from build123d import *

# Parameters (mm, degrees)
SKETCH014_R          = 2.2
PAD013_DEPTH         = 1.8
SKETCH015_W          = 30
SKETCH015_H          = 6
PAD014_DEPTH         = 0.75
FILLET004_R          = 0.7499
SKETCH016_W          = 25
SKETCH016_H          = 15
SKETCH017_W          = 6.5
SKETCH017_H          = 15
LOFT_PLACEMENT_ANGLE = 180
PAD015_DEPTH         = 3.25
SKETCH019_R          = 1.75
POCKET003_DEPTH      = 6.5


with BuildPart() as fillet004:
    # Sketch014 → Pad013 (new body)
    with BuildSketch(Plane.XZ):
        with BuildLine():
            Line((-25.5, 7.5), (25.5, 7.5))
            ThreePointArc((27.5, 5.5), (26.914214, 6.914214), (25.5, 7.5))
            Line((27.5, 5.5), (27.5, -5.5))
            ThreePointArc((25.5, -7.5), (26.914214, -6.914214), (27.5, -5.5))
            Line((25.5, -7.5), (-25.5, -7.5))
            ThreePointArc((-27.5, -5.5), (-26.914214, -6.914214), (-25.5, -7.5))
            Line((-27.5, -5.5), (-27.5, 5.5))
            ThreePointArc((-25.5, 7.5), (-26.914214, 6.914214), (-27.5, 5.5))
        make_face()
        with Locations((-20, 0)):
            Circle(SKETCH014_R, mode=Mode.SUBTRACT)
        with Locations((20, 0)):
            Circle(SKETCH014_R, mode=Mode.SUBTRACT)
    extrude(amount=PAD013_DEPTH)

    # Sketch015 → Pad014 (new body)
    with BuildSketch(Plane.XZ.offset(1.8)):
        Rectangle(SKETCH015_W, SKETCH015_H)
    extrude(amount=PAD014_DEPTH)

    # Fillet004
    fillet004_edges = [fillet004.edges().sort_by_distance(p)[0] for p in [
        (-15, -2.55, 0),
        (0, -2.55, 3),
        (15, -2.55, 0),
        (0, -2.55, -3),
    ]]
    fillet(fillet004_edges, radius=FILLET004_R)


with BuildPart() as fusion001:
    # Sketch016 → Loft section 0
    with BuildSketch(Plane.XZ):
        Rectangle(SKETCH016_W, SKETCH016_H)
    # Sketch017 → Loft section 1
    with BuildSketch(Plane.XZ.offset(15)):
        Rectangle(SKETCH017_W, SKETCH017_H)
    loft(ruled=True)


with BuildPart() as fusion001_1:
    # Loft placement: moved
    add(fusion001.part.rotate(Axis((0, 0, 0), (0, 0, 1)), LOFT_PLACEMENT_ANGLE))

    # Fusion001: union Fillet004
    add(fillet004.part)


with BuildPart() as fusion002:
    # Sketch018 → Pad015 (new body, symmetric)
    with BuildSketch(Plane(origin=(0, 15, 0), x_dir=(0, 1, 0), z_dir=(1, 0, 0))):
        with BuildLine():
            Line((0, 7.5), (9, 7.5))
            ThreePointArc((9, -7.5), (16.5, 0), (9, 7.5))
            Line((9, -7.5), (0, -7.5))
            Line((0, -7.5), (0, 7.5))
        make_face()
    extrude(amount=PAD015_DEPTH, both=True)

    # Sketch019 → Pocket003 (cut)
    with BuildSketch(Plane(origin=(3.25, 15, 0), x_dir=(0, 1, 0), z_dir=(1, 0, 0))):
        with Locations((9, 0)):
            Circle(SKETCH019_R)
    extrude(amount=-POCKET003_DEPTH, mode=Mode.SUBTRACT)

    # Fusion002: union Fusion001
    add(fusion001_1.part)


solid = fusion002.part
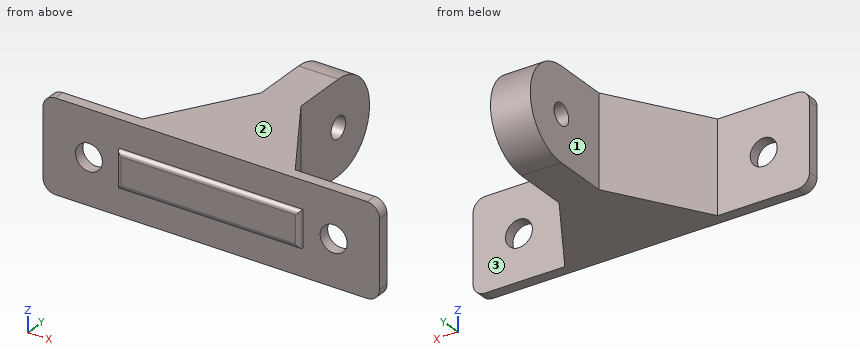
Can you work these out from the model? Positions are in its coordinate system, mm. Face numbers are marked on the shaded views. A direction names the side the tool comes from. Round coordinates to 2 decimals unless told otherwise and drop trailing zeros. Order: outer loops, then holes, each group sorted by start corner. A loop starts at its lowest first (then second) coordinate and runs counter-clockwise, first axis right, second up. Notation, with made-up numbers: (-37.75, -9.75) -> (-13.75, -9.75) arc R25 ccw to (-13.75, 5.25) -> close; hole circle Ø1 at (-28.75, -29). An arc over 180 degrees is marked (long way). Write each question's results on one line, items separated by ' | '. Start each with the question number.
Item 1: If we section it at A-A, the plane z = 0: State how many separate pieces and enclosed holes the cut face has, then the cut area to 3 significant figures.
Item 2: Please list where these lines run through material, in increasing order: L1, parallel to Z at x = 2, y = 24; L2, parallel to Y at x = -14, z = -0.5; L3, parallel to X at y = 25.5, z = -5.75.
Item 3: Will these pins go through, and if not, where does the flat tip stop? pin 1 (5 mm diameter, centred on x = 20, z = 0, fed in from -Y); pin 2 (4 mm diameter, centred on y = 24, z = 0, fed in from +X); pin 3 (7.5 mm diameter, centred on x = 23.5, z = 3.5, fed in from +Y).
Item 4: Which directions (+Z, -Z, +X, -X, +Y, -Y) give clear straight access to the entire face, cutting with the end or side of a thin tool? Please do the marked faces 1, 2 and 3.
Item 5: If we section it at B-B, the plane x = -20: Write out the boundary of the cut face in (y, z), then the cut area to 3 significant figures.
Results:
1) separate pieces: 4 | enclosed holes: 0 | area: 426 mm2
2) L1: z = -7.5 to -1.75, 1.75 to 7.5 | L2: y = -2.55 to 0 | L3: x = -3.25 to 3.25
3) pin 1: stops at y = -1.8 | pin 2: stops at x = 3.25 | pin 3: stops at y = 0
4) face 1: +Z, -Z, -X, +Y | face 2: +Z, +X, -X, +Y, -Y | face 3: +Z, -Z, +X, +Y
5) outline: (-1.8, -7.5) -> (0, -7.5) -> (0, -2.2) -> (-1.8, -2.2) -> close; (-1.8, 2.2) -> (0, 2.2) -> (0, 7.5) -> (-1.8, 7.5) -> close | area: 19.1 mm2
